Model file for the job. Use its own axes, mm. A direction names the side the tool comes from. Coordinates: 2 decimals unless noted, no trailing zeros. Order: outer loops, then holes, each group sorted by start corner. A loop starts at its lowest first (then second) coordinate and runs counter-clockwise, first axis right, second up. Notation, with made-up numbers: (20.25, 38.25) - (46.25, 38.25) arc R27 ccw to (46.25, 71.25) - close; hole circle Ø11 at (-1, -27.5). An arc over 180 degrees is marked (long way). Put each result on its own line as item: value. Start each with the question number.
```python
from build123d import *

# Parameters (mm, degrees)
BOSS_EXTRUDE1_DEPTH     = 17
CUT_EXTRUDE1_DEPTH      = 44
CUT_EXTRUDE1_DEPTH_BACK = 15
SKETCH3_W               = 9.47
SKETCH3_H               = 10.75
CUT_EXTRUDE2_REACH      = 25.642
SKETCH5_W               = 10
SKETCH5_H               = 10.75
SKETCH6_R               = 4
CUT_EXTRUDE3_DEPTH      = 20


with BuildPart() as part:
    # Sketch1 → Boss-Extrude1 (new body)
    with BuildSketch(Plane.XY):
        Polygon((-16.550185094, 16.389351475), (-16.550185094, 1.389351475), (-10.343680533, -14.570648525), (-4.883984447, -18.349711721), (11.8091046, -3.684474659), (13.567850846, 1.389351475), (13.567850846, 16.389351475), (8.527850846, 16.389351475), (8.527850846, 5.292351475), (-11.510185094, 5.292351475), (-11.510185094, 16.389351475), align=None)
    extrude(amount=BOSS_EXTRUDE1_DEPTH)

    # Sketch2 → Cut-Extrude1 (cut, two sides)
    with BuildSketch(Plane(origin=(-11.510185094, 0, 0), x_dir=(0, 0, -1), z_dir=(1, 0, 0))) as cut_extrude1_sk:
        with BuildLine():
            Line((-17, 16.389351475), (-17, 5.292351475))
            ThreePointArc((-17, 5.292351475), (-14.707938783, 12.187976499), (-8.743930787, 16.339337446))
            Line((-8.743930787, 16.339337446), (-3.743930787, 15.776730228))
            Line((-3.743930787, 15.776730228), (0, 12.052351475))
            Line((0, 12.052351475), (0, 16.389351475))
            Line((0, 16.389351475), (-17, 16.389351475))
        make_face()
    extrude(amount=CUT_EXTRUDE1_DEPTH, mode=Mode.SUBTRACT)
    extrude(cut_extrude1_sk.sketch, amount=-CUT_EXTRUDE1_DEPTH_BACK, mode=Mode.SUBTRACT)

    # Cut-Sweep1: sweep along a path in Sketch4
    with BuildLine(Plane(origin=(0, 0, 10), x_dir=(-1, 0, 0), z_dir=(0, 0, -1))) as cut_sweep1_path:
        Line((0.820338721, -14.779711721), (9.490783662, -9.250648525))
    # Sketch3 → Cut-Sweep1 (sweep, cut)
    with BuildSketch(Plane(origin=(6.970965598, -7.934883628, 0), x_dir=(0.751264134, 0.660001668, 0), z_dir=(0.660001668, -0.751264134, 0))):
        with Locations((-7.025002686, 7.885)):
            Rectangle(SKETCH3_W, SKETCH3_H)
    sweep(path=cut_sweep1_path.line, mode=Mode.SUBTRACT)

    # Cut-Extrude2: up to this face of the body (flat: up to its plane)
    cut_extrude2_end = Plane(part.part.faces().sort_by_distance((-6.1991251, -12.931973418, 7.885))[0])
    # Sketch5 → Cut-Extrude2 (cut, up to the picked face)
    with BuildSketch(Plane(origin=(0, 5.292351475, 0), x_dir=(1, 0, 0), z_dir=(0, 1, 0)), mode=Mode.PRIVATE) as cut_extrude2_sk1:
        with Locations((0.107850846, -7.885)):
            Rectangle(SKETCH5_W, SKETCH5_H)
    cut_extrude2_tool1 = split(extrude(cut_extrude2_sk1.sketch, amount=-CUT_EXTRUDE2_REACH, mode=Mode.PRIVATE), bisect_by=cut_extrude2_end, keep=Keep.BOTH, mode=Mode.PRIVATE)
    add(cut_extrude2_tool1.solids().sort_by_distance((0.107851, 5.292351, 7.885))[0], mode=Mode.SUBTRACT)

    # Sketch6 → Cut-Extrude3 (cut, symmetric)
    with BuildSketch(Plane(origin=(-1.491167124, 0, 0), x_dir=(0, 0, -1), z_dir=(1, 0, 0))):
        with Locations((-8.5, 9.989351475)):
            Circle(SKETCH6_R)
    extrude(amount=CUT_EXTRUDE3_DEPTH, both=True, mode=Mode.SUBTRACT)


solid = part.part
```
Item 1: Pull direction X, two halves, no side cores. Call faces 3 (the face through (-13.49, -6.48, 8.38)), 4 (the face through (-7.67, -7.65, 7.81)), 5 (the face through (-11.51, 8.3, 4.6)), 6 (the face through (12.676, -1.183, 8.381)): pulls with the +X half, pulls with the -X half, needs draft (parallel to the pull), parting line crosses it, or undercut.
Item 2: Wall check: line 1 along X through (y, z) = (2, 4); line 2 along X through (y, z) = (9.5, 3.75); line 3 along Y through (x, z) = (-10, 5). Give the ranges that are in metal, low to high.
Item 3: 3-axis set-ups, long thin cutter, end or side, ignore diameter. For faces 1 (the face through (11.013, 16.062, 6.279)), 2 (the face through (-6.26, -12.893, 7.96)): which of +Z, -Z, +X, -X, +Y, -Y reach the whole face in a straight line?
Item 4: Slice it at B-B, the plane x = 2. Give the cut face in (y, z), plus the area to 3 significant figures.
Item 5: Slice it at C-C, the plane z = 10.25. Give the cut face in (x, y).
Item 6: Slice it at A-A, the plane y = 2. Give the cut face in (x, z).
Item 7: Flat gauge pins, fed straight in: pin 1 Ø8.5 at (x, z) = (3.5, 10.5) entering from +Y; pin 2 Ø8.5 at (y, z) = (-4.5, 10) entering from -X; pin 3 Ø10 at (y, z) = (-5, 12.5) entering from +X. Where does each tip first touch, or does it go through?
Item 8: Slice it at D-D, the plane x = -13. Give the cut face in (y, z).
Here are the results:
1. face 3: pulls with the -X half
1. face 4: undercut
1. face 5: undercut
1. face 6: pulls with the +X half
2. line 1: x = -16.55 to -4.89, 5.11 to 13.57
2. line 2: x = -16.55 to -11.51, 8.53 to 13.57
2. line 3: y = -14.81 to -10.51, -9.7 to 5.29
3. face 1: -Z, +X, -X, +Y
3. face 2: +X
4. outline: (-12.3, 0) - (5.29, 0) - (5.29, 2.51) - (-12.3, 2.51) - close; (-12.3, 13.26) - (5.29, 13.26) - (5.29, 17) - (-12.3, 17) - close
4. area: 110 mm^2
5. outline: (-16.55, 1.39) - (-10.34, -14.57) - (-4.88, -18.35) - (-1.86, -15.7) - (-10.53, -10.17) - (-4.89, -5.21) - (-4.89, 5.29) - (-11.51, 5.29) - (-11.51, 6.39) - (-16.55, 6.39) - close; (-16.55, 13.59) - (-11.51, 13.59) - (-11.51, 15.78) - (-16.55, 15.78) - close; (5.11, -9.36) - (5.25, -9.45) - (11.81, -3.68) - (13.57, 1.39) - (13.57, 6.39) - (8.53, 6.39) - (8.53, 5.29) - (5.11, 5.29) - close; (8.53, 13.59) - (13.57, 13.59) - (13.57, 15.78) - (8.53, 15.78) - close
6. outline: (-16.55, 0) - (13.57, 0) - (13.57, 17) - (-16.55, 17) - close; hole (-4.89, 2.51) - (5.11, 2.51) - (5.11, 13.26) - (-4.89, 13.26) - close
7. pin 1: stops at y = 5.29
7. pin 2: stops at x = -15.91
7. pin 3: stops at x = 13.09
8. outline: (-7.74, 0) - (12.05, 0) - (15.78, 3.74) - (16.34, 8.74) arc R11.52 ccw to (5.29, 17) - (-7.74, 17) - close; hole circle Ø8 at (9.99, 8.5)
